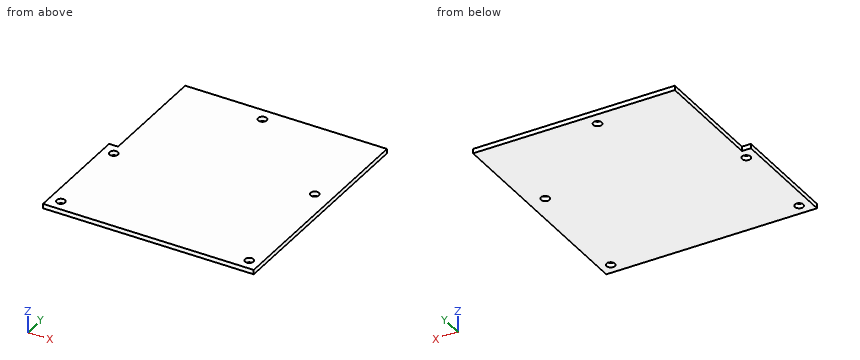
```python
from build123d import *

# Parameters (mm, degrees)
SKETCH1_R           = 1.5
BOSS_EXTRUDE1_DEPTH = 1.6002


with BuildPart() as part:
    # Sketch1 → Boss-Extrude1 (new body)
    with BuildSketch(Plane.XY):
        Polygon((74.93, 80.645), (3.175, 80.645), (3.175, 40.005), (0, 40.005), (0, 0), (74.93, 0), align=None)
        with Locations((68.984, 47.026)):
            Circle(SKETCH1_R, mode=Mode.SUBTRACT)
        with Locations((33.3595, 76.026)):
            Circle(SKETCH1_R, mode=Mode.SUBTRACT)
        with Locations((3.984, 36.026)):
            Circle(SKETCH1_R, mode=Mode.SUBTRACT)
        with Locations((70.984, 4.026)):
            Circle(SKETCH1_R, mode=Mode.SUBTRACT)
        with Locations((3.984, 4.026)):
            Circle(SKETCH1_R, mode=Mode.SUBTRACT)
    extrude(amount=BOSS_EXTRUDE1_DEPTH)


solid = part.part
```
The listing builds one solid part. Answer for the finished solid, in the listing's coordinates (mm). Give positions to 0.01 mm unless a question says otherwise; leave off trailing zeros. Order: outer loops, then holes, each group sorted by start corner. A loop starts at its lowest first (then second) coordinate and runs counter-clockwise, first axis right, second up.
1) Find section A-A on z = 0.75. Write down the section's boundary in (x, y) (1 decimal).
Reported:
outline: (0, 0) - (74.9, 0) - (74.9, 80.6) - (3.2, 80.6) - (3.2, 40) - (0, 40) - close; hole circle Ø3 at (4, 4); hole circle Ø3 at (4, 36); hole circle Ø3 at (33.4, 76); hole circle Ø3 at (69, 47); hole circle Ø3 at (71, 4)
2) Given P1, Ø0.5, axis at y = 62.5, z = 0.5, coming from the -X side (3 decimals), flat-ended and moving along its own axis, determine where the tip first touches the part or whether it passes through.
Reported:
P1: stops at x = 3.175
3) Consider line 1 along Y through (x, z) = (33.5, 0.8) (3 decimals); line 2 along Y through (x, z) = (32, 1.2) (3 decimals); line 3 along X through (y, z) = (57, 1.05) (3 decimals). Determine where each line is inside the solid, lowest interval first.
Reported:
line 1: y = 0 to 74.533, 77.519 to 80.645
line 2: y = 0 to 75.392, 76.66 to 80.645
line 3: x = 3.175 to 74.93
4) Find section B-B on y = 53.5. Write down the section's boundary in (x, z) (3 decimals), then the cut area to 3 significant figures.
Reported:
outline: (3.175, 0) - (74.93, 0) - (74.93, 1.6) - (3.175, 1.6) - close
area: 115 mm2
